Geometry check sheet. Reference: the model listing, model coordinates, mm. Face numbers are marked on the shaded views. A direction names the side the tool comes from. Coordinates: 2 decimals unless noted, no trailing zeros. Write each loop counter-clockwise with the first axis right and the second up, starting at its lowest first coordinate (ties: lowest second). Pieces come first, ordered by that corner, then holes. Notation, with made-up numbers: M 35.25,19.25 L 69.25,19.25 A11 cw 69.25,32.25 Z; hole C 67.25,88 d10. An arc over 180 degrees is marked long. Answer as a JSON object with one key per item and string values. Group by question number.
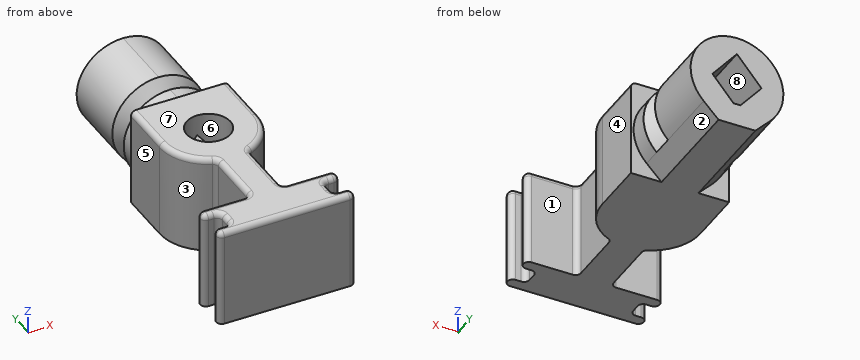
```python
from build123d import *

# Parameters (mm, degrees)
F0_R      = 4
F1_DEPTH  = 18
F3_R      = 0.99999
F6_DEPTH  = 20
F8_DEPTH  = 30
F9_SIZE   = 1
F10_R     = 5
F11_DEPTH = 3.5


# Not quite as in the source:
# - two fillets or chamfers of one size are made in one step
# - a fillet or chamfer is up to 0.001 mm smaller than in the source, because OpenCascade refuses the exact size


with BuildPart() as f1:
    # F0 (on Top) → F1 (new body)
    with BuildSketch(Plane.XY):
        with BuildLine():
            Line((3, -20), (3, -8.4852813742))
            ThreePointArc((3, -8.4852813742), (7.3484692283, -5.1961524227), (9, 0))
            Line((9, 0), (9, 30))
            Line((9, 30), (-9, 30))
            Line((-9, 30), (-9, 0))
            ThreePointArc((-9, 0), (-7.3484692283, -5.1961524227), (-3, -8.4852813742))
            Line((-3, -8.4852813742), (-3, -20))
            Line((-3, -20), (-12.5, -20))
            Line((-12.5, -20), (-12.5, -22))
            Line((-12.5, -22), (-9.5, -22))
            Line((-9.5, -22), (-9.5, -25.6))
            Line((-9.5, -25.6), (-12.5, -25.6))
            Line((-12.5, -25.6), (-12.5, -27.6))
            Line((-12.5, -27.6), (0, -27.6))
            Line((0, -27.6), (12.5, -27.6))
            Line((12.5, -27.6), (12.5, -25.6))
            Line((12.5, -25.6), (9.5, -25.6))
            Line((9.5, -25.6), (9.5, -22))
            Line((9.5, -22), (12.5, -22))
            Line((12.5, -22), (12.5, -20))
            Line((12.5, -20), (3, -20))
        make_face()
        Circle(F0_R, mode=Mode.SUBTRACT)
    extrude(amount=F1_DEPTH)

    # F3 (radius 1 in the source; OpenCascade refuses exactly that, so slightly less here)
    f3_edges = [f1.edges().sort_by_distance(p)[0] for p in [
        (3, -20, 9),
        (-3, -20, 9),
        (3, -8.485281, 9),
        (12.5, -27.6, 9),
        (-12.5, -27.6, 9),
        (-9.5, -25.6, 9),
        (-12.5, -25.6, 9),
        (-9.5, -22, 9),
        (-12.5, -22, 9),
        (-12.5, -20, 9),
        (12.5, -25.6, 9),
        (9.5, -25.6, 9),
        (9.5, -22, 9),
        (12.5, -22, 9),
        (12.5, -20, 9),
        (3, -14.242641, 18),
        (7.348469, -5.196152, 18),
        (9, 15, 18),
        (-9, 15, 18),
        (-7.348469, -5.196152, 18),
        (-3, -14.242641, 18),
        (-7.75, -20, 18),
        (-12.5, -21, 18),
        (-11, -22, 18),
        (-9.5, -23.8, 18),
        (-11, -25.6, 18),
        (-12.5, -26.6, 18),
        (0, -27.6, 18),
        (12.5, -26.6, 18),
        (11, -25.6, 18),
        (9.5, -23.8, 18),
        (11, -22, 18),
        (12.5, -21, 18),
        (7.75, -20, 18),
        (-3, -8.485281, 9),
    ]]
    fillet(f3_edges, radius=F3_R)

    # F5 (on face) → F6 (cut)
    with BuildSketch(Plane(origin=(0, 30, 0), x_dir=(-1, 0, 0), z_dir=(0, 1, 0))):
        with BuildLine():
            Line((-11.1393053085, 0), (-9, 0))
            Line((-9, 0), (-9, 17.00001))
            ThreePointArc((-9, 17.00001), (-8.7071097101, 17.7071097101), (-8.00001, 18))
            Line((-8.00001, 18), (8.00001, 18))
            ThreePointArc((8.00001, 18), (8.7071097101, 17.7071097101), (9, 17.00001))
            Line((9, 17.00001), (9, 21.8532588333))
            Line((9, 21.8532588333), (-11.1393053085, 21.8532588333))
            Line((-11.1393053085, 21.8532588333), (-11.1393053085, 0))
        make_face()
        with BuildLine():
            Line((6.1143883029, 2.836985475), (3.3747432753, 0))
            Line((3.3747432753, 0), (9, 0))
            Line((9, 0), (9, 17.00001))
            ThreePointArc((9, 17.00001), (8.7071097101, 17.7071097101), (8.00001, 18))
            Line((8.00001, 18), (-8.00001, 18))
            ThreePointArc((-8.00001, 18), (-8.7071097101, 17.7071097101), (-9, 17.00001))
            Line((-9, 17.00001), (-9, 0))
            Line((-9, 0), (-3.3747432753, 0))
            Line((-3.3747432753, 0), (-6.1143883029, 2.836985475))
            ThreePointArc((-6.1143883029, 2.836985475), (-7.8242912543, 12.0627962161), (0, 17.2415816239))
            ThreePointArc((0, 17.2415816239), (7.8242912543, 12.0627962161), (6.1143883029, 2.836985475))
        make_face()
    extrude(amount=-F6_DEPTH, mode=Mode.SUBTRACT)

    # F7 (on face) → F8 (cut)
    with BuildSketch(Plane(origin=(0, 30, 0), x_dir=(-1, 0, 0), z_dir=(0, 1, 0))):
        Polygon((4.5, 8.7415816239), (0, 14.1044727906), (-4.5, 8.7415816239), (0, 3.3786904573), align=None)
    extrude(amount=-F8_DEPTH, mode=Mode.SUBTRACT)

    # F9
    f9_edges = [f1.edges().sort_by_distance(p)[0] for p in [
        (0, 17, 3.37869),
    ]]
    chamfer(f9_edges, length=F9_SIZE)

    # F10 (on face) → F11 (join)
    with BuildSketch(Plane(origin=(0, 0, 0), x_dir=(1, 0, 0), z_dir=(0, 0, -1))):
        Circle(F10_R)
    extrude(amount=-F11_DEPTH)

    # F12 (on Right) → F13 (revolve, cut)
    with BuildSketch(Plane.YZ):
        Polygon((17.5, 17.2415816239), (13.5, 17.2415816239), (15.5, 15.2415816239), align=None)
    revolve(axis=Axis((0, 30, 8.7415816239), (0, 1, 0)), mode=Mode.SUBTRACT)


solid = f1.part
```
1) Section check C-C (y = -16). Record the cut outline in (x, z).
2) Section check D-D (y = 3). Record the cut outline in (x, z), then the cut area to 3 significant figures.
3) Section check A-A (y = 24.5). Record the cut outline in (x, z), then the cut area to 3 significant figures.
4) Draft check along X on the marked faces 5, 6, 7 and 8. Enter one of: +X half, -X half, draft (parallel to the pull), parting line (faces both ways), or undercut.
5) Material ranges on probe 1 along Y at (x, z) = (0, 14.5); probe 2 along X at (y, z) = (0, 14.5); probe 3 along Z at (x, y) = (0.25, 17), recorded low to high. Write a range as [from, to].
6) Set-up check for the marked faces 1, 2, 3 and 4: record each of +Z, -Z, +X, -X, +Y, -Y from which the full face is reachable in a straight line by a thin tool's end or side.
7) Section check B-B (x = 7.25). State how many separate pieces and enclosed holes the cut face has, then the cut area to 3 significant figures.
8) Go/stop test with flat-tipped pins: pin 1 Ø5 at (x, z) = (-7.5, 3) entering from +Y; pin 2 Ø0.5 at (x, z) = (-11, 6.5) entering from +Y; pin 3 Ø2.5 at (x, y) = (-0.5, 1) entering from +Z; pin 4 Ø0.8 at (y, z) = (-24, 9.5) entering from -X. Record where each tip stops, or that it passes through.
Entries:
{
 "1": {"outline": "M -3,0 L 3,0 L 3,17 A1 ccw 2,18 L -2,18 A1 ccw -3,17 Z"},
 "2": {"outline": "M -9,0 L 9,0 L 9,17 A1 ccw 8,18 L 2.65,18 L 2.65,10.95 L 4.5,8.74 L 2.65,6.53 L 2.65,3.5 L -2.65,3.5 L -2.65,6.53 L -4.5,8.74 L -2.65,10.95 L -2.65,18 L -8,18 A1 ccw -9,17 Z", "area": "239 mm^2"},
 "3": {"outline": "M -6.11,2.84 L -3.37,0 L 3.37,0 L 6.11,2.84 A8.5 ccw long Z; hole M -4.5,8.74 L -0.64,4.14 L 0.64,4.14 L 4.5,8.74 L 0,14.1 Z", "area": "184 mm^2"},
 "4": {"face 5": "-X half", "face 6": "undercut", "face 7": "draft", "face 8": "undercut"},
 "5": {"probe 1": "[-27.6, -4], [4, 30]", "probe 2": "[-9, -4], [4, 9]", "probe 3": "[0, 0.25], [0.75, 4.14], [13.81, 16.74]"},
 "6": {"face 1": "+Z, -Z, +X", "face 2": "-Z, +X, +Y", "face 3": "+Z, -Z, -X", "face 4": "+Z, -Z, +X, +Y"},
 "7": {"separate pieces": "3", "enclosed holes": "0", "area": "569 mm^2"},
 "8": {"pin 1": "y = 30", "pin 2": "y = -20", "pin 3": "z = 3.5", "pin 4": "x = -9.5"}
}
